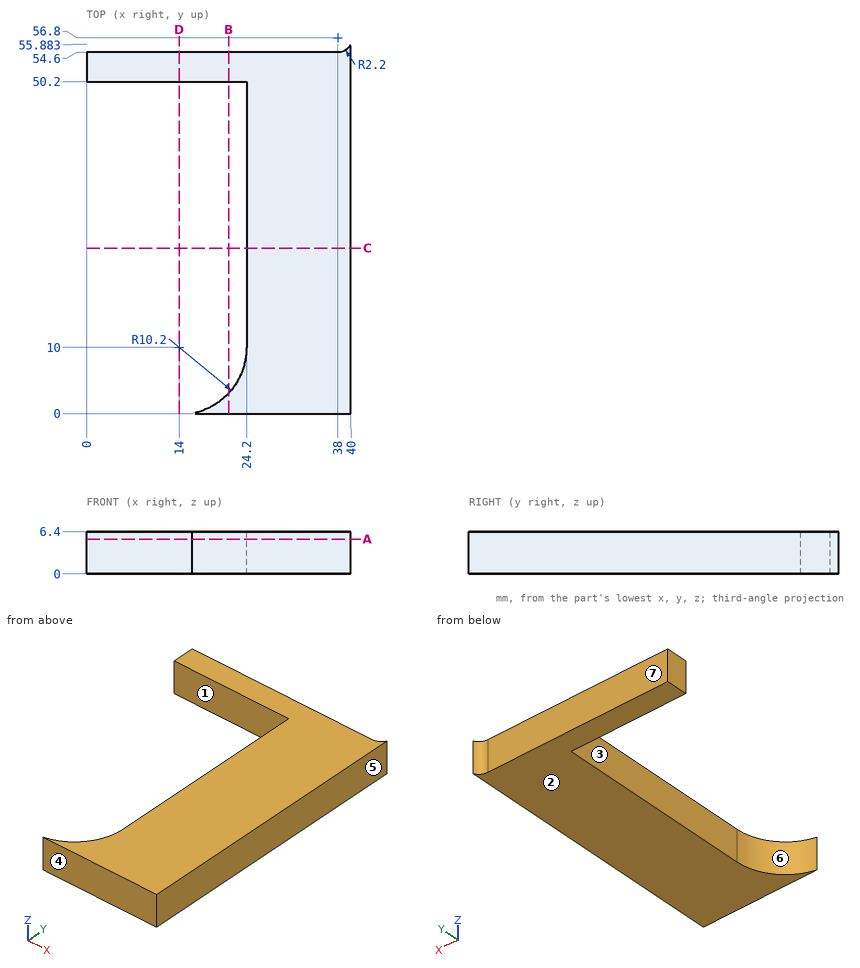
Can you work these out from the drawing? Everything is in mm from the part's minimum corner. A direction names the side the tool comes from. Give positions to 0.01 mm unless a question says otherwise; leave off trailing zeros. Order: outer loops, then holes, each group sorted by start corner. A loop starts at its lowest first (then second) coordinate and runs counter-clockwise, first axis right, second up. Notation, with made-up numbers: M 74,0 L 132,0 A16 cw 132,20 Z; hole C 18.25,-16 d2. An arc over 180 degrees is marked long. Use a Markdown table: item, result. Add a question column.
Item 1: Suppose I cut it at A-A (z = 5.25). List the corners of the cut face in (x, y) for me.
Item 2: Suppose I cut it at D-D (x = 14). List the corners of the cut face in (y, z) for me.
Item 3: Suppose I cut it at C-C (y = 25). List the corners of the cut face in (x, z) for me.
Item 4: If I drill on L1, parallel to X at y = 23.5, z = 3.75; L2, parallel to Y at x = 33, z = 1; L3, parallel to Y at x = 7.5, z = 6.25, over which ranges is the centre line in solid material (lowest first)? Write a range as [from, to].
Item 5: We'd pull the mould along Y, two halves only. Please class the marked faces 1, 2, 3 and 4: +Y half, -Y half, draft (parallel to the pull), parting line (faces both ways), or undercut.
Item 6: Will these pins go through, and if not, where does the flat tip stop? pin 1 (3 mm diameter, centred on x = 24.5, z = 1.5, fed in from -Y); pin 2 (1.9 mm diameter, centred on x = 14.5, z = 2, fed in from +Y).
Item 7: For the marked faces 5, 6 and 7, which set-ups out of +Z, -Z, +X, -X, +Y, -Y let a thin tool reach every point of the face, with its end or its side?
Item 8: Suppose I cut it at B-B (x = 21.5). List the corners of the cut face in (y, z) for me.
Answer sheet:
| question | item | result |
|---|---|---|
| 1 | outline | M 0,50.2 L 24.2,50.2 L 24.2,10 A10.2 cw 16.01,0 L 40,0 L 40,55.88 A2.2 cw 38,54.6 L 0,54.6 Z |
| 2 | outline | M 50.2,0 L 54.6,0 L 54.6,6.4 L 50.2,6.4 Z |
| 3 | outline | M 24.2,0 L 40,0 L 40,6.4 L 24.2,6.4 Z |
| 4 | L1 | x = [24.2, 40] |
| 4 | L2 | y = [0, 54.6] |
| 4 | L3 | y = [50.2, 54.6] |
| 5 | face 1 | undercut |
| 5 | face 2 | draft |
| 5 | face 3 | undercut |
| 5 | face 4 | -Y half |
| 6 | pin 1 | stops at y = 0 |
| 6 | pin 2 | stops at y = 54.6 |
| 7 | face 5 | +Z, -Z, +X, +Y, -Y |
| 7 | face 6 | +Z, -Z, -X |
| 7 | face 7 | +Z, -Z, -X, +Y |
| 8 | outline | M 0,0 L 3.09,0 L 3.09,6.4 L 0,6.4 Z; M 50.2,0 L 54.6,0 L 54.6,6.4 L 50.2,6.4 Z |
